from build123d import *

# Parameters (mm, degrees)
BOSS_EXTRUDE1_DEPTH             = 10
SKETCH2_W                       = 8
SKETCH2_H                       = 4.2
CUT_EXTRUDE1_DEPTH              = 4
SKETCH3_W                       = 8
SKETCH3_H                       = 4
BOSS_EXTRUDE2_DEPTH             = 4
SKETCH4_W                       = 14
SKETCH4_H                       = 4
CUT_EXTRUDE2_DEPTH              = 109.5
CIRPATTERN4_COUNT               = 5
CIRPATTERN4_ANGLE               = 72
CIRPATTERN4_THE_OTHER_WAY_COUNT = 5
CIRPATTERN4_THE_OTHER_WAY_ANGLE = 72


with BuildPart() as part:
    # Sketch1 → Boss-Extrude1 (new body)
    with BuildSketch(Plane(origin=(0, 0, 0), x_dir=(1, 0, 0), z_dir=(0, 1, 0))):
        with BuildLine():
            Line((-4, 112.5), (-4, 108.426242211))
            ThreePointArc((-4, 108.426242211), (-93.963756311, 54.25), (-95.899880192, -50.74901949))
            Line((-95.899880192, -50.74901949), (-99.427857926, -52.785898385))
            Line((-99.427857926, -52.785898385), (-97.427857926, -56.25))
            Line((-97.427857926, -56.25), (-91.365680099, -52.75))
            ThreePointArc((-91.365680099, -52.75), (-91.365680099, 52.75), (0, 105.5))
            Line((0, 105.5), (0, 112.5))
            Line((0, 112.5), (-4, 112.5))
        make_face()
    extrude(amount=BOSS_EXTRUDE1_DEPTH)

    # Sketch2 → Cut-Extrude1 (cut)
    with BuildSketch(Plane(origin=(-97.427857926, 0, 56.25), x_dir=(0.5, 0, 0.866025404), z_dir=(-0.866025404, 0, 0.5))):
        with Locations((0, 5)):
            Rectangle(SKETCH2_W, SKETCH2_H)
    extrude(amount=-CUT_EXTRUDE1_DEPTH, mode=Mode.SUBTRACT)

    # Sketch3 → Boss-Extrude2 (add)
    with BuildSketch(Plane(origin=(0, 0, -112.5), x_dir=(-1, 0, 0), z_dir=(0, 0, -1))):
        with Locations((0, 5)):
            Rectangle(SKETCH3_W, SKETCH3_H)
    extrude(amount=-BOSS_EXTRUDE2_DEPTH)

    # Sketch4 → Cut-Extrude2 (cut, through all)
    with BuildSketch(Plane(origin=(0, 0, 0), x_dir=(0, 0, -1), z_dir=(1, 0, 0))):
        with Locations((-9.672320837, 5)):
            Rectangle(SKETCH4_W, SKETCH4_H)
    cut_extrude2 = extrude(amount=-CUT_EXTRUDE2_DEPTH, mode=Mode.SUBTRACT)

    # CirPattern4: Cut-Extrude2 ×5 about axis
    cirpattern4_axis = Axis((0, 0, 0), (0, -1, 0))
    for i in range(1, CIRPATTERN4_COUNT):
        add(cut_extrude2.rotate(cirpattern4_axis, i * CIRPATTERN4_ANGLE / (CIRPATTERN4_COUNT - 1)), mode=Mode.SUBTRACT)

    # CirPattern4 the other way: Cut-Extrude2 ×5 about axis
    cirpattern4_the_other_way_axis = Axis((0, 0, 0), (0, 1, 0))
    for i in range(1, CIRPATTERN4_THE_OTHER_WAY_COUNT):
        add(cut_extrude2.rotate(cirpattern4_the_other_way_axis, i * CIRPATTERN4_THE_OTHER_WAY_ANGLE / (CIRPATTERN4_THE_OTHER_WAY_COUNT - 1)), mode=Mode.SUBTRACT)


solid = part.part
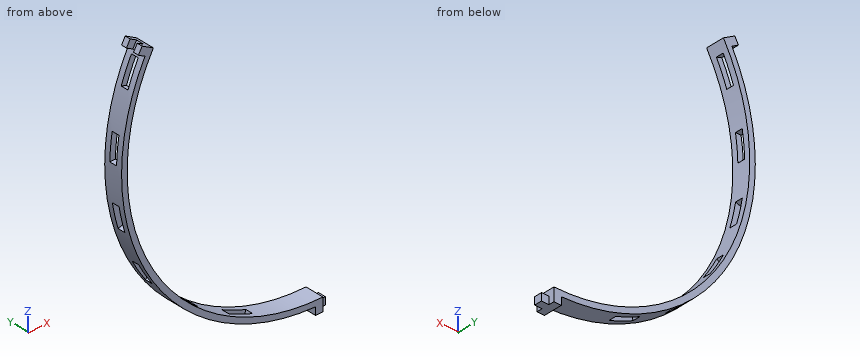
For this review, take the finished solid that the model builds, in its own axes (mm). Coordinates: 2 decimals unless noted, no trailing zeros. Loops run counter-clockwise (first coordinate to the right, second up) from the corner with the lowest first, then second, coordinate; pieces in that order, holes last. Notation, with made-up numbers: (86, 73) - (114, 73) arc R27 ccw to (114, 111) - close; hole circle Ø4 at (75.5, -13.5). An arc over 180 degrees is marked (long way). Use a Markdown table: item, result. Add a question column.
Item 1: For line 1 (Z direction, x = -2, y = 3.5); line 2 (X direction, y = 8.75, z = -30.5); line 3 (X direction, y = 7.5, z = -59), list the stretches that pass through material, from the lowest coordinate up.
Item 2: We need section A-A (y = 5.5). Give the number of separate pieces and of enclosed holes in the cut face, and give its area (3 significant figures).
Item 3: We need section B-B (x = -28.5). Give the boundary of the cut face in (y, z), and give its area (3 significant figures).
Item 4: We need section C-C (z = 24.5). Give the boundary of the cut face in (x, y).
Item 5: Insertion check: pin 1 Ø1 at (x, y) = (-93, 5.5) entering from -Z; pin 2 Ø2 at (y, z) = (7.5, -111.5) entering from -X; pin 3 Ø2 at (x, z) = (2, -110) entering from +Y. Each pin has a flat end and moves straight along its axis. Give the tip position at first contact, or say it passes through.
Results list:
| question | item | result |
|---|---|---|
| 1 | line 1 | z = -112.5 to -105.48 |
| 1 | line 2 | x = -104.12 to -101 |
| 1 | line 3 | x = -91.06 to -87.46 |
| 2 | separate pieces | 7 |
| 2 | enclosed holes | 0 |
| 2 | area | 451 mm^2 |
| 3 | outline | (0, -104.69) - (10, -104.69) - (10, -101.58) - (0, -101.58) - close |
| 3 | area | 31.1 mm^2 |
| 4 | outline | (-105.7, 0) - (-102.62, 0) - (-102.62, 10) - (-105.7, 10) - close |
| 5 | pin 1 | stops at z = 48.87 |
| 5 | pin 2 | stops at x = -4 |
| 5 | pin 3 | stops at y = 7 |
